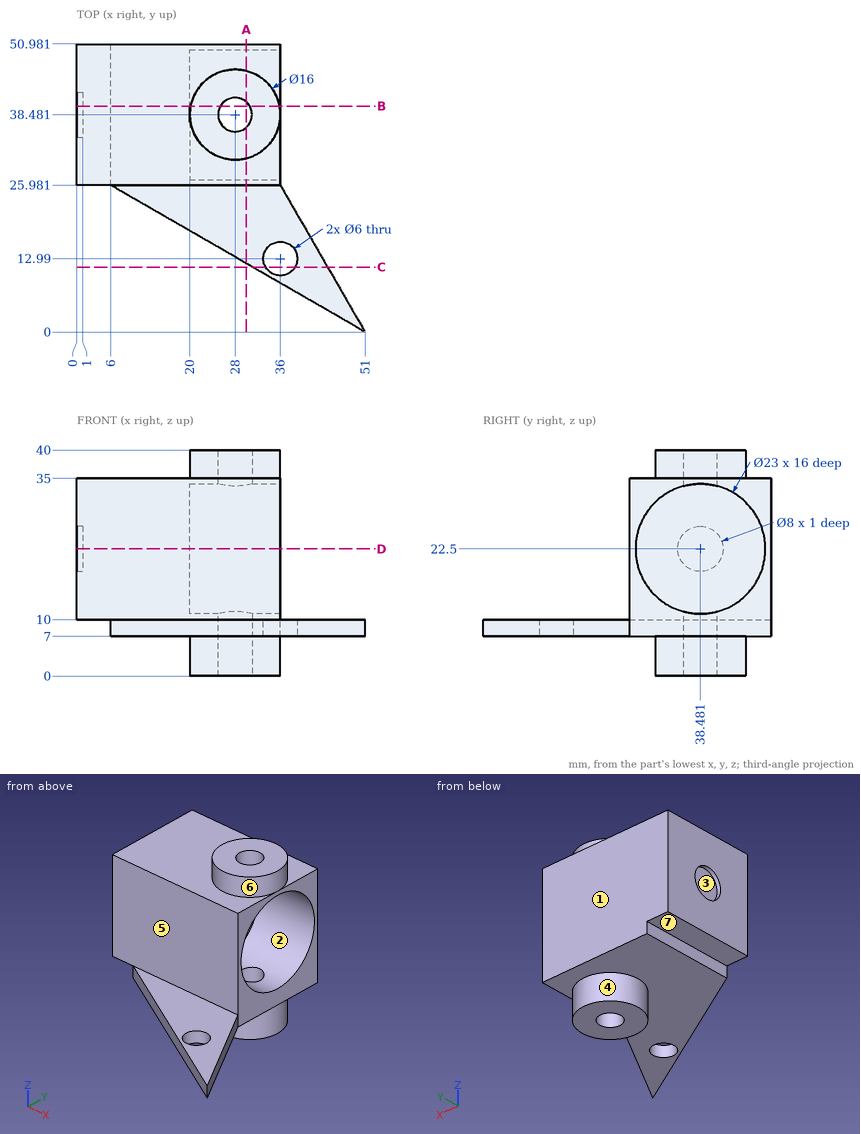
Answer from the drawing. Dimensions are ordinates in mm from the lowest x, y and z of the part. A direction names the side the tool comes from. Coordinates: 2 decimals unless noted, no trailing zeros. Loops run counter-clockwise (first coordinate to the right, second up) from the corner with the lowest first, then second, coordinate; pieces in that order, holes last. Notation, with made-up numbers: (82.25, 71.25) - (109.25, 71.25) arc R25 ccw to (109.25, 110.25) - close; hole circle Ø8 at (3.25, -26). An arc over 180 degrees is marked (long way). Answer in a Markdown table with one row per item.
1. Straight lines are drawn through the part: line 1 (Y direction, x = 28, z = 2.75); line 2 (Y direction, x = 24, z = 22); line 3 (X direction, y = 32.5, z = 17). For each, find the intervals that lie inside material, in ascending order.
Conclusion:
| item | result |
|---|---|
| line 1 | y = 30.48 to 35.48, 41.48 to 46.48 |
| line 2 | y = 25.98 to 26.99, 49.97 to 50.98 |
| line 3 | x = 0 to 20 |
2. Find section A-A, the plane x = 30. Write down the section's boundary in (y, z) (1 decimal).
Conclusion:
| item | result |
|---|---|
| outline | (12.1, 7) - (30.7, 7) - (30.7, 0) - (36.2, 0) - (36.2, 11.2) arc R11.5 cw to (36.2, 33.8) - (36.2, 40) - (30.7, 40) - (30.7, 35) - (26, 35) - (26, 10) - (12.1, 10) - close; (40.7, 0) - (46.2, 0) - (46.2, 7) - (51, 7) - (51, 35) - (46.2, 35) - (46.2, 40) - (40.7, 40) - (40.7, 33.8) arc R11.5 cw to (40.7, 11.2) - close |
3. Determine the mould class of the marked faces 1, 2, 3 and 4 for opening direction Y: +Y half, -Y half, draft (parallel to the pull), parting line (faces both ways), or undercut.
Conclusion:
| item | result |
|---|---|
| face 1 | +Y half |
| face 2 | undercut |
| face 3 | undercut |
| face 4 | parting line |
4. Find section D-D, the plane z = 22.5. Write down the section's boundary in (x, y), then the cut area to 3 significant figures.
Conclusion:
| item | result |
|---|---|
| outline | (0, 25.98) - (36, 25.98) - (36, 26.98) - (20, 26.98) - (20, 49.98) - (36, 49.98) - (36, 50.98) - (0, 50.98) - (0, 42.48) - (1, 42.48) - (1, 34.48) - (0, 34.48) - close |
| area | 524 mm² |
5. Given pin 1 (9.5 mm diameter, centred on x = 36, y = 12.99, fed in from -Z); pin 2 (4 mm diameter, centred on x = 19.5, z = 13.5, fed in from -Y); pin 3 (18.5 mm diameter, centred on y = 41, z = 27, fed in from +X), each flat-ended and moving along its own axis, determine where each tip first touches the part or whether it passes through.
Conclusion:
| item | result |
|---|---|
| pin 1 | stops at z = 7 |
| pin 2 | stops at y = 25.98 |
| pin 3 | stops at x = 36 |
6. Which of the six approach directions +Z, -Z, +X, -X, +Y, -Y give full straight-line access (tool end or side, diameter ignored) to the marked faces 5, 6 and 7?
Conclusion:
| item | result |
|---|---|
| face 5 | +Z, +X, -X, -Y |
| face 6 | +Z |
| face 7 | -Z, -X, +Y, -Y |
7. Find section C-C, the plane y = 11.5. Write down the section's boundary in (x, z), then the cut area to 3 significant figures.
Conclusion:
| item | result |
|---|---|
| outline | (31.08, 7) - (33.4, 7) - (33.4, 10) - (31.08, 10) - close; (38.6, 7) - (44.36, 7) - (44.36, 10) - (38.6, 10) - close |
| area | 24.2 mm² |
8. Find section B-B, the plane y = 40. Count the separate pieces of the cut face and the enclosed holes in it, then the cut area to 3 significant figures.
Conclusion:
| item | result |
|---|---|
| separate pieces | 3 |
| enclosed holes | 0 |
| area | 717 mm² |
